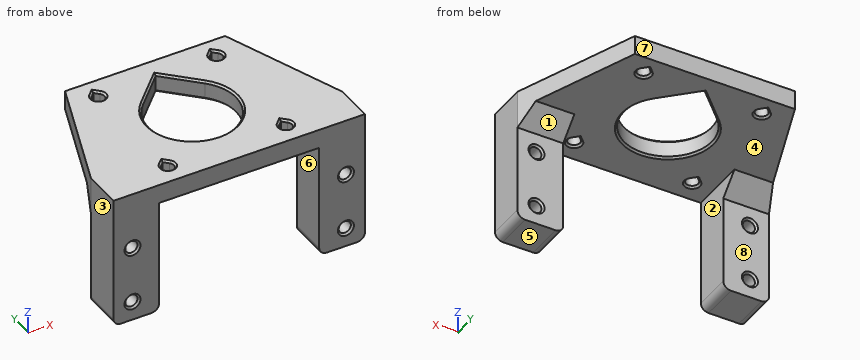
```python
from build123d import *

# Parameters (mm, degrees)
EXTRUDE_1_DEPTH     = 5
SKETCH_2_W          = 12
SKETCH_2_H          = 10
EXTRUDE_2_DEPTH     = 30
EXTRUDE_3_DEPTH     = 5
SKETCH_5_R          = 1.6
CUT_EXTRUDE_1_DEPTH = 55.890800686
FILLET_1_R          = 2
CHAMFER_1_SIZE      = 5
CHAMFER_2_SIZE      = 0.5


with BuildPart() as part:
    # 草图1 → 凸台-拉伸1 (new body)
    with BuildSketch(Plane.XY):
        Polygon((-21, 21), (21, 21), (21, -11), (33, -11), (33, -21), (-33, -21), (-33, -11), (-21, -11), align=None)
        with BuildLine():
            Line((-15.5, 17.7627417), (-16.63137085, 16.63137085))
            ThreePointArc((-16.63137085, 16.63137085), (-15.5, 13.9), (-14.36862915, 16.63137085))
            Line((-14.36862915, 16.63137085), (-15.5, 17.7627417))
        make_face(mode=Mode.SUBTRACT)
        with BuildLine():
            Line((-15.5, -13.2372583), (-16.63137085, -14.36862915))
            ThreePointArc((-16.63137085, -14.36862915), (-15.5, -17.1), (-14.36862915, -14.36862915))
            Line((-14.36862915, -14.36862915), (-15.5, -13.2372583))
        make_face(mode=Mode.SUBTRACT)
        with BuildLine():
            Line((-8.131727984, 8.131727984), (0, 16.263455967))
            Line((0, 16.263455967), (8.131727984, 8.131727984))
            ThreePointArc((8.131727984, 8.131727984), (0, -11.5), (-8.131727984, 8.131727984))
        make_face(mode=Mode.SUBTRACT)
        with BuildLine():
            Line((15.5, -13.2372583), (14.36862915, -14.36862915))
            ThreePointArc((14.36862915, -14.36862915), (15.5, -17.1), (16.63137085, -14.36862915))
            Line((16.63137085, -14.36862915), (15.5, -13.2372583))
        make_face(mode=Mode.SUBTRACT)
        with BuildLine():
            Line((15.5, 17.7627417), (14.36862915, 16.63137085))
            ThreePointArc((14.36862915, 16.63137085), (15.5, 13.9), (16.63137085, 16.63137085))
            Line((16.63137085, 16.63137085), (15.5, 17.7627417))
        make_face(mode=Mode.SUBTRACT)
    extrude(amount=EXTRUDE_1_DEPTH)

    # 草图2 → 凸台-拉伸2 (add)
    with BuildSketch(Plane(origin=(0, 0, 0), x_dir=(-1, 0, 0), z_dir=(0, 0, -1))):
        with Locations((-27, -16)):
            Rectangle(SKETCH_2_W, SKETCH_2_H)
        with Locations((27, -16)):
            Rectangle(SKETCH_2_W, SKETCH_2_H)
    extrude(amount=EXTRUDE_2_DEPTH)

    # 草图3 → 凸台-拉伸3 (add)
    with BuildSketch(Plane.XY.offset(5)):
        Polygon((-21, 21), (-33, -11), (-21, -11), align=None)
        Polygon((21, -11), (21, 21), (33, -11), align=None)
    extrude(amount=-EXTRUDE_3_DEPTH)

    # 草图5 → 切除-拉伸1 (cut, through all)
    with BuildSketch(Plane(origin=(0, -11, 0), x_dir=(1, 0, 0), z_dir=(0, 1, 0))):
        with Locations(Location((28, 25, 0), (0, 0, 270))):
            Circle(SKETCH_5_R)
        with Locations(Location((28, 10, 0), (0, 0, 270))):
            Circle(SKETCH_5_R)
        with Locations(Location((-28, 10, 0), (0, 0, 270))):
            Circle(SKETCH_5_R)
        with Locations(Location((-28, 25, 0), (0, 0, 270))):
            Circle(SKETCH_5_R)
    extrude(amount=-CUT_EXTRUDE_1_DEPTH, mode=Mode.SUBTRACT)

    # 圆角1
    fillet_1_edges = [part.edges().sort_by_distance(p)[0] for p in [
        (33, -16, -30),
        (21, -16, -30),
        (-21, -16, -30),
        (-33, -16, -30),
    ]]
    fillet(fillet_1_edges, radius=FILLET_1_R)

    # 倒角1
    chamfer_1_edges = [part.edges().sort_by_distance(p)[0] for p in [
        (-27, -11, 0),
        (27, -11, 0),
    ]]
    chamfer(chamfer_1_edges, length=CHAMFER_1_SIZE)

    # 倒角2
    chamfer_2_edges = [part.edges().sort_by_distance(p)[0] for p in [
        (-28, -21, -26.6),
        (-28, -11, -26.6),
        (-28, -21, -11.6),
        (-28, -11, -11.6),
        (28, -21, -11.6),
        (28, -11, -11.6),
        (28, -21, -26.6),
        (28, -11, -26.6),
        (0, -11.5, 0),
        (4.065863992, 12.197591975, 0),
        (-4.065863992, 12.197591975, 0),
        (0, -11.5, 5),
        (4.065863992, 12.197591975, 5),
        (-4.065863992, 12.197591975, 5),
        (-15.5, -17.1, 0),
        (-14.934314575, -13.802943725, 0),
        (-16.065685425, -13.802943725, 0),
        (-15.5, -17.1, 5),
        (-14.934314575, -13.802943725, 5),
        (-16.065685425, -13.802943725, 5),
        (-15.5, 13.9, 0),
        (-14.934314575, 17.197056275, 0),
        (-16.065685425, 17.197056275, 0),
        (-15.5, 13.9, 5),
        (-14.934314575, 17.197056275, 5),
        (-16.065685425, 17.197056275, 5),
        (16.065685425, 17.197056275, 0),
        (14.934314575, 17.197056275, 0),
        (15.5, 13.9, 0),
        (16.065685425, 17.197056275, 5),
        (14.934314575, 17.197056275, 5),
        (15.5, 13.9, 5),
        (15.5, -17.1, 0),
        (16.065685425, -13.802943725, 0),
        (14.934314575, -13.802943725, 0),
        (15.5, -17.1, 5),
        (16.065685425, -13.802943725, 5),
        (14.934314575, -13.802943725, 5),
    ]]
    chamfer(chamfer_2_edges, length=CHAMFER_2_SIZE)


solid = part.part
```
Build history of the part. All positions in model axes, mm. Face numbers are marked on the shaded views. A direction names the side the tool comes from. Give positions to 0.01 mm unless a question says otherwise; leave off trailing zeros. Loops run counter-clockwise (first coordinate to the right, second up) from the corner with the lowest first, then second, coordinate; pieces in that order, holes last.
1) Band-saw the part on A-A on y = -15.5. State how many separate pieces and enclosed holes the cut face has, then the cut area to 3 significant figures.
Values follow:
separate pieces: 3
enclosed holes: 4
area: 981 mm2
2) Band-saw the part on B-B on z = -10. List the corners of the cut face in (x, y).
Values follow:
outline: (-33, -21) - (-30.1, -21) - (-29.6, -20.5) - (-29.6, -11.5) - (-30.1, -11) - (-33, -11) - close; (-26.4, -20.5) - (-25.9, -21) - (-21, -21) - (-21, -11) - (-25.9, -11) - (-26.4, -11.5) - close; (21, -21) - (25.9, -21) - (26.4, -20.5) - (26.4, -11.5) - (25.9, -11) - (21, -11) - close; (29.6, -20.5) - (30.1, -21) - (33, -21) - (33, -11) - (30.1, -11) - (29.6, -11.5) - close
3) Two-plate mould, pull along X, no slides. Class the marked faces 1, 2 and 3: released by +X, released by -X, zero draft, split by the parting line, or undercut.
Values follow:
face 1: zero draft
face 2: undercut
face 3: released by -X
4) Band-saw the part on D-D on z = -15. List the corners of the cut face in (x, y).
Values follow:
outline: (-33, -21) - (-21, -21) - (-21, -11) - (-33, -11) - close; (21, -21) - (33, -21) - (33, -11) - (21, -11) - close
5) Drop flat-ended pins along their axis: P1, Ø3.5, axis at x = -28, z = -10, coming from the -Y side; P2, Ø21, axis at x = -12, y = 4, coming from the -Z side; P3, Ø9.5, axis at x = 24.5, z = -12, coming from the +Y side. Give the stop position or say it passes through.
Values follow:
P1: stops at y = -20.65
P2: stops at z = 0
P3: stops at y = -11
6) 3-axis set-ups, long thin cutter, end or side, ignore diameter. For the marked faces 4, 5, 6, 7 and 8: which of +Z, -Z, +X, -X, +Y, -Y reach the whole face in a straight line?
Values follow:
face 4: -Z, +Y
face 5: -Z, +X, -X, +Y, -Y
face 6: -Z, +Y, -Y
face 7: +Z, -Z, +X, -X, +Y
face 8: -Z, +X, -X, +Y
7) Band-saw the part on C-C on x = -28. List the corners of the cut face in (y, z).
Values follow:
outline: (-21, -30) - (-11, -30) - (-11, -27.1) - (-11.5, -26.6) - (-20.5, -26.6) - (-21, -27.1) - close; (-21, -22.9) - (-20.5, -23.4) - (-11.5, -23.4) - (-11, -22.9) - (-11, -12.1) - (-11.5, -11.6) - (-20.5, -11.6) - (-21, -12.1) - close; (-21, -7.9) - (-20.5, -8.4) - (-11.5, -8.4) - (-11, -7.9) - (-11, -5) - (-6, 0) - (2.33, 0) - (2.33, 5) - (-21, 5) - close
8) Probe line 1 along X through (y, z) = (-14.5, -25); line 2 along X through (y, z) = (-13.5, -24.5); line 3 along Z through (x, y) = (27, -17.5). List the from-to ranges inside material, lowest first.
Values follow:
line 1: x = -33 to -29.6, -26.4 to -21, 21 to 26.4, 29.6 to 33
line 2: x = -33 to -29.52, -26.48 to -21, 21 to 26.48, 29.52 to 33
line 3: z = -30 to -26.25, -23.75 to -11.25, -8.75 to 5
